from build123d import *

# Parameters (mm, degrees)
SKETCH_1_W          = 42
SKETCH_1_H          = 42
EXTRUDE_1_DEPTH     = 59
SKETCH_2_R          = 11
EXTRUDE_2_DEPTH     = 2
SKETCH_3_R          = 2.5
EXTRUDE_3_DEPTH     = 21
CUT_EXTRUDE_START   = -8
CUT_EXTRUDE_1_DEPTH = 42
CHAMFER_1_SIZE      = 4


with BuildPart() as part:
    # 草图1 → 凸台-拉伸1 (new body)
    with BuildSketch(Plane(origin=(0, 0, 0), x_dir=(0, 0, -1), z_dir=(1, 0, 0))):
        Rectangle(SKETCH_1_W, SKETCH_1_H)
    extrude(amount=EXTRUDE_1_DEPTH)

    # 草图2 → 凸台-拉伸2 (add)
    with BuildSketch(Plane(origin=(59, 0, 0), x_dir=(0, 0, -1), z_dir=(1, 0, 0))):
        Circle(SKETCH_2_R)
    extrude(amount=EXTRUDE_2_DEPTH)

    # 草图3 → 凸台-拉伸3 (add)
    with BuildSketch(Plane(origin=(61, 0, 0), x_dir=(0, 0, -1), z_dir=(1, 0, 0))):
        with Locations(Location((0, 0, 0), (0, 0, 180))):
            Circle(SKETCH_3_R)
    extrude(amount=EXTRUDE_3_DEPTH)

    # 草图5 → 切除-拉伸1 (cut)
    with BuildSketch(Plane.ZY.offset(CUT_EXTRUDE_START)):
        Polygon((21, 15), (15, 21), (21, 21), align=None)
        Polygon((21, -21), (21, -15), (15, -21), align=None)
        Polygon((-21, 21), (-21, 15), (-15, 21), align=None)
        Polygon((-21, -15), (-15, -21), (-21, -21), align=None)
    extrude(amount=-CUT_EXTRUDE_1_DEPTH, mode=Mode.SUBTRACT)

    # 倒角1
    chamfer_1_edges = [part.edges().sort_by_distance(p)[0] for p in [
        (4, 21, 21),
        (4, 21, -21),
        (4, -21, -21),
        (4, -21, 21),
        (54.5, 21, 21),
        (54.5, 21, -21),
        (54.5, -21, -21),
        (54.5, -21, 21),
    ]]
    chamfer(chamfer_1_edges, length=CHAMFER_1_SIZE)


solid = part.part
CAD build for the part. Positions are in the model's coordinates, mm. A direction names the side the tool comes from. Give positions to 0.01 mm unless a question says otherwise; leave off trailing zeros. Loops run counter-clockwise (first coordinate to the right, second up) from the corner with the lowest first, then second, coordinate; pieces in that order, holes last. Notation, with made-up numbers: M -1,66.5 L 36,66.5 A14 ccw 36,74.5 Z; hole C 26,32.25 d5. An arc over 180 degrees is marked long. One line per question, with ' | ' between items. Start each with the question number.
1. Saw through at A-A on y = 0. Give the cut face in (x, z).
2. 3-axis set-ups, long thin cutter, end or side, ignore diameter. For faces 1 (the face through (50, 18.5, 18.2)), 2 (the face through (29, 18, -18)), 3 (the face through (71.4, -0.1, -2.5)): which of +Z, -Z, +X, -X, +Y, -Y reach the whole face in a straight line?
3. Probe L1, parallel to X at y = 13.5, z = 13.5; L2, parallel to X at y = 6, z = -4; L3, parallel to Y at x = 67, z = 0.5. List the from-to ranges inside material, lowest first. Write a range as from..to.
4. Saw through at B-B on x = 48. Give the cut face in (y, z).
5. Flat gauge pins, fed straight in: pin 1 (6.5 mm diameter, centred on y = 19.5, z = -18.5, fed in from +X); pin 2 (5 mm diameter, centred on y = 7, z = 9.5, fed in from +X). Where does each tip first touch, or does it go through?
6. Saw through at D-D on y = 13. Give the cut face in (x, z).
Result sheet:
1) outline: M 0,-21 L 59,-21 L 59,-11 L 61,-11 L 61,-2.5 L 82,-2.5 L 82,2.5 L 61,2.5 L 61,11 L 59,11 L 59,21 L 0,21 Z
2) face 1: +Z, +Y | face 2: -Z, +Y | face 3: +X
3) L1: x = 0..59 | L2: x = 0..61 | L3: y = -2.45..2.45
4) outline: M -21,-15 L -15,-21 L 15,-21 L 21,-15 L 21,15 L 15,21 L -15,21 L -21,15 Z
5) pin 1: stops at x = 59 | pin 2: stops at x = 61
6) outline: M 0,-21 L 59,-21 L 59,21 L 0,21 Z
